```python
from build123d import *

# Parameters (mm, degrees)
F0_R     = 3.302
F0_R_2   = 4.7625
F1_DEPTH = 4.064
F3_DEPTH = 19.05
F4_DEPTH = 11.0871
F6_DEPTH = 6.35


with BuildPart() as f1:
    # F0 (on Top) → F1 (new body)
    with BuildSketch(Plane.XY):
        with BuildLine():
            ThreePointArc((-10.8559225607, -3.7088047495), (-25.0461002864, -34.6422404521), (-29.9085, -68.326))
            Line((-29.9085, -68.326), (-29.9085, -101.346))
            ThreePointArc((-29.9085, -101.346), (-28.7925768363, -104.0400768363), (-26.0985, -105.156))
            Line((-26.0985, -105.156), (0, -105.156))
            Line((0, -105.156), (26.0985, -105.156))
            ThreePointArc((26.0985, -105.156), (28.7925768363, -104.0400768363), (29.9085, -101.346))
            Line((29.9085, -101.346), (29.9085, -68.326))
            ThreePointArc((29.9085, -68.326), (25.0461002864, -34.6422404521), (10.8559225607, -3.7088047495))
            ThreePointArc((10.8559225607, -3.7088047495), (8.4291493536, -1.3414386781), (5.215684606, -0.2610245767))
            ThreePointArc((5.215684606, -0.2610245767), (2.6111060749, -0.0652969534), (0, 0))
            ThreePointArc((0, 0), (-2.6111060749, -0.0652969534), (-5.215684606, -0.2610245767))
            ThreePointArc((-5.215684606, -0.2610245767), (-8.4291493536, -1.3414386781), (-10.8559225607, -3.7088047495))
        make_face()
        with Locations((-19.2405, -82.931)):
            Circle(F0_R, mode=Mode.SUBTRACT)
        with Locations((19.2405, -82.931)):
            Circle(F0_R, mode=Mode.SUBTRACT)
        with Locations((0, -51.562)):
            Circle(F0_R_2, mode=Mode.SUBTRACT)
        with Locations((0, -17.4625)):
            Circle(F0_R, mode=Mode.SUBTRACT)
    extrude(amount=F1_DEPTH)

    # F2 (on Right) → F3 (join, symmetric)
    with BuildSketch(Plane.YZ):
        with BuildLine():
            Line((-51.6255, 4.064), (-32.5755, 4.064))
            ThreePointArc((-32.5755, 4.064), (-36.4801215826, 5.7092093226), (-38.0299678542, 9.6526545109))
            ThreePointArc((-38.0299678542, 9.6526545109), (-38.3159932296, 10.1220079213), (-38.8616980577, 10.0563620532))
            ThreePointArc((-38.8616980577, 10.0563620532), (-42.1005, 8.89), (-45.3393019423, 10.0563620532))
            ThreePointArc((-45.3393019423, 10.0563620532), (-45.8850067704, 10.1220079213), (-46.1710321458, 9.6526545109))
            ThreePointArc((-46.1710321458, 9.6526545109), (-47.7208784174, 5.7092093226), (-51.6255, 4.064))
        make_face()
    extrude(amount=F3_DEPTH, both=True)

    # F2 (on Right) → F4 (cut, symmetric)
    with BuildSketch(Plane.YZ):
        with BuildLine():
            Line((-51.6255, 4.064), (-32.5755, 4.064))
            ThreePointArc((-32.5755, 4.064), (-36.4801215826, 5.7092093226), (-38.0299678542, 9.6526545109))
            ThreePointArc((-38.0299678542, 9.6526545109), (-38.3159932296, 10.1220079213), (-38.8616980577, 10.0563620532))
            ThreePointArc((-38.8616980577, 10.0563620532), (-42.1005, 8.89), (-45.3393019423, 10.0563620532))
            ThreePointArc((-45.3393019423, 10.0563620532), (-45.8850067704, 10.1220079213), (-46.1710321458, 9.6526545109))
            ThreePointArc((-46.1710321458, 9.6526545109), (-47.7208784174, 5.7092093226), (-51.6255, 4.064))
        make_face()
    extrude(amount=F4_DEPTH, both=True, mode=Mode.SUBTRACT)

    # F5 (on Top) → F6 (join)
    with BuildSketch(Plane.XY):
        with BuildLine():
            ThreePointArc((5.4185637479, 1.7608221173), (0, 2.032), (-5.4185637479, 1.7608221173))
            ThreePointArc((-5.4185637479, 1.7608221173), (-9.4889524281, 0.3922975888), (-12.5628651572, -2.6063661016))
            ThreePointArc((-12.5628651572, -2.6063661016), (-26.9951425328, -34.067559391), (-31.9405, -68.326))
            Line((-31.9405, -68.326), (-31.9405, -101.346))
            ThreePointArc((-31.9405, -101.346), (-30.2294178157, -105.4769178157), (-26.0985, -107.188))
            Line((-26.0985, -107.188), (26.0985, -107.188))
            ThreePointArc((26.0985, -107.188), (30.2294178157, -105.4769178157), (31.9405, -101.346))
            Line((31.9405, -101.346), (31.9405, -68.326))
            ThreePointArc((31.9405, -68.326), (26.9951425328, -34.067559391), (12.5628651572, -2.6063661016))
            ThreePointArc((12.5628651572, -2.6063661016), (9.4889524281, 0.3922975888), (5.4185637479, 1.7608221173))
        make_face()
        with BuildLine():
            ThreePointArc((-29.9085, -68.326), (-25.0461002864, -34.6422404521), (-10.8559225607, -3.7088047495))
            ThreePointArc((-10.8559225607, -3.7088047495), (-8.4291493536, -1.3414386781), (-5.215684606, -0.2610245767))
            ThreePointArc((-5.215684606, -0.2610245767), (0, 0), (5.215684606, -0.2610245767))
            ThreePointArc((5.215684606, -0.2610245767), (8.4291493536, -1.3414386781), (10.8559225607, -3.7088047495))
            ThreePointArc((10.8559225607, -3.7088047495), (25.0461002864, -34.6422404521), (29.9085, -68.326))
            Line((29.9085, -68.326), (29.9085, -101.346))
            ThreePointArc((29.9085, -101.346), (28.7925768363, -104.0400768363), (26.0985, -105.156))
            Line((26.0985, -105.156), (-26.0985, -105.156))
            ThreePointArc((-26.0985, -105.156), (-28.7925768363, -104.0400768363), (-29.9085, -101.346))
            Line((-29.9085, -101.346), (-29.9085, -68.326))
        make_face(mode=Mode.SUBTRACT)
    extrude(amount=F6_DEPTH)


solid = f1.part
```
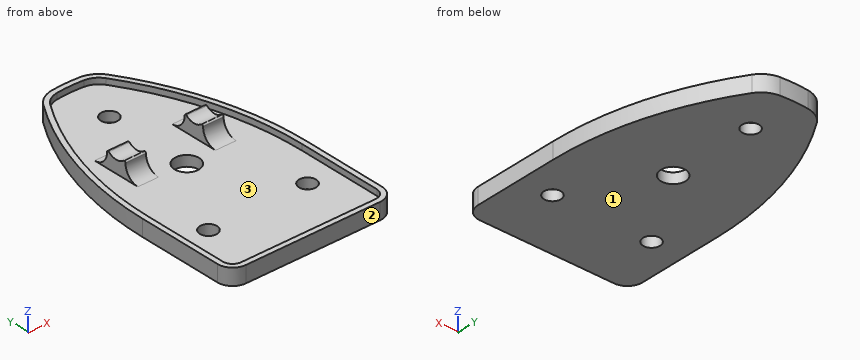
CAD build for the part. Positions are in the model's coordinates, mm. Face numbers are marked on the shaded views. Give positions to 0.01 mm unless a question says otherwise; leave off trailing zeros. Loops run counter-clockwise (first coordinate to the right, second up) from the corner with the lowest first, then second, coordinate; pieces in that order, holes last. Notation, with made-up numbers: (88, -11.5) - (111, -11.5) arc R34 ccw to (111, 23.5) - close; hole circle Ø2 at (75, 14.5). An arc over 180 degrees is marked (long way). Put each result on its own line as item: value.
Q1. Probe line 1 along Y through (x, z) = (0, 2.5); line 2 along Z through (x, y) = (-12, -66); line 3 along Y through (x, z) = (-19.5, 4.5). List the from-to ranges inside material, lowest first.
Filled in:
line 1: y = -107.19 to -56.32, -46.8 to -20.76, -14.16 to 2.03
line 2: z = 0 to 4.06
line 3: y = -107.19 to -105.16, -19.63 to -14.85
Q2. Slice it at A-A (x = 0). Give the cut face in (y, z), plus the area to 3 significant figures.
Filled in:
outline: (-107.19, 0) - (-56.32, 0) - (-56.32, 4.06) - (-105.16, 4.06) - (-105.16, 6.35) - (-107.19, 6.35) - close; (-46.8, 0) - (-20.76, 0) - (-20.76, 4.06) - (-46.8, 4.06) - close; (-14.16, 0) - (2.03, 0) - (2.03, 6.35) - (0, 6.35) - (0, 4.06) - (-14.16, 4.06) - close
area: 388 mm²
Q3. Slice it at C-C (y = -67). Give the cut face in (x, z), plus the area to 3 significant figures.
Filled in:
outline: (-31.93, 0) - (31.93, 0) - (31.93, 6.35) - (29.9, 6.35) - (29.9, 4.06) - (-29.9, 4.06) - (-29.9, 6.35) - (-31.93, 6.35) - close
area: 269 mm²
Q4. Slice it at D-D (y = -22.5). Give the cut face in (x, z).
Filled in:
outline: (-22.94, 0) - (22.94, 0) - (22.94, 6.35) - (20.74, 6.35) - (20.74, 4.06) - (-20.74, 4.06) - (-20.74, 6.35) - (-22.94, 6.35) - close
Q5. Mould opens along Z. For the marked faces 1, 2 and 3 say: pulls with the +Z half, pulls with the -Z half, needs draft (parallel to the pull), parting line crosses it, or undercut.
Filled in:
face 1: pulls with the -Z half
face 2: needs draft
face 3: pulls with the +Z half
Q6. Slice it at B-B (x = -21.5). Give the cut face in (y, z), plus the area to 3 significant figures.
Filled in:
outline: (-107.19, 0) - (-85.34, 0) - (-85.34, 4.06) - (-105.16, 4.06) - (-105.16, 6.35) - (-107.19, 6.35) - close; (-80.52, 0) - (-19.13, 0) - (-19.13, 6.35) - (-24.37, 6.35) - (-24.37, 4.06) - (-80.52, 4.06) - close
area: 355 mm²
Q7. Flat gauge pins, fed straight in: pin 1 (1.8 mm diameter, centred on y = -47, z = 8.5, fed in from -X); pin 2 (5 mm diameter, centred on y = -21.5, z = 4, fed in from -X); pin 3 (1.5 mm diameter, centred on x = -19, y = -48, fed in from +Z). Where does each tip first touch, or does it go through?
Filled in:
pin 1: stops at x = -19.05
pin 2: stops at x = -23.54
pin 3: stops at z = 6.26
